```python
from build123d import *

# Parameters (mm, degrees)
SKETCH3_W           = 20
SKETCH3_H           = 60
BOSS_EXTRUDE3_DEPTH = 5
CUT_EXTRUDE2_DEPTH  = 2
SKETCH6_R           = 3.57
CUT_EXTRUDE3_DEPTH  = 3
SKETCH7_W           = 20
SKETCH7_H           = 10
BOSS_EXTRUDE4_DEPTH = 17.5
SKETCH8_R           = 2.1
CUT_EXTRUDE4_DEPTH  = 40
SKETCH9_W           = 1.25
SKETCH9_H           = 25
CUT_EXTRUDE5_DEPTH  = 30


with BuildPart() as part:
    # Sketch3 → Boss-Extrude3 (new body)
    with BuildSketch(Plane.XY):
        Rectangle(SKETCH3_W, SKETCH3_H)
    extrude(amount=BOSS_EXTRUDE3_DEPTH)

    # Sketch4 → Cut-Extrude2 (cut)
    with BuildSketch(Plane.XY.offset(5)):
        with BuildLine():
            Line((-2.85, 19.850023256), (-1.875, 7.739206809))
            Line((-1.875, 7.739206809), (1.875, 7.739206809))
            Line((1.875, 7.739206809), (2.85, 19.850023256))
            ThreePointArc((2.85, 19.850023256), (0, 18.43), (-2.85, 19.850023256))
        make_face()
        with BuildLine():
            Line((1.875, 7.739206809), (-1.875, 7.739206809))
            ThreePointArc((-1.875, 7.739206809), (0, 5.864206809), (1.875, 7.739206809))
        make_face()
        with BuildLine():
            ThreePointArc((3.57, 22), (-1.133666618, 25.385217866), (-2.85, 19.850023256))
            Line((-2.85, 19.850023256), (2.85, 19.850023256))
            ThreePointArc((2.85, 19.850023256), (3.385217866, 20.866333382), (3.57, 22))
        make_face()
        with BuildLine():
            Line((2.85, 19.850023256), (-2.85, 19.850023256))
            ThreePointArc((-2.85, 19.850023256), (0, 18.43), (2.85, 19.850023256))
        make_face()
    extrude(amount=-CUT_EXTRUDE2_DEPTH, mode=Mode.SUBTRACT)

    # Sketch6 → Cut-Extrude3 (cut)
    with BuildSketch(Plane.XY.offset(3)):
        with Locations((0, 22)):
            Circle(SKETCH6_R)
    extrude(amount=-CUT_EXTRUDE3_DEPTH, mode=Mode.SUBTRACT)

    # Sketch7 → Boss-Extrude4 (add)
    with BuildSketch(Plane(origin=(0, 0, 0), x_dir=(-1, 0, 0), z_dir=(0, 0, -1))):
        with Locations((0, -25)):
            Rectangle(SKETCH7_W, SKETCH7_H)
    extrude(amount=BOSS_EXTRUDE4_DEPTH)

    # Sketch8 → Cut-Extrude4 (cut)
    with BuildSketch(Plane(origin=(0, 0, -17.5), x_dir=(-1, 0, 0), z_dir=(0, 0, -1))):
        with Locations((0, -25)):
            Circle(SKETCH8_R)
    extrude(amount=-CUT_EXTRUDE4_DEPTH, mode=Mode.SUBTRACT)

    # Sketch9 → Cut-Extrude5 (cut)
    with BuildSketch(Plane(origin=(10, 0, 0), x_dir=(0, 0, -1), z_dir=(1, 0, 0))):
        with Locations((-0.625, 17.5)):
            Rectangle(SKETCH9_W, SKETCH9_H)
    extrude(amount=-CUT_EXTRUDE5_DEPTH, mode=Mode.SUBTRACT)


solid = part.part
```
Here's how the part is built. I have some questions about the finished solid (model axes, mm). A direction names the side the tool comes from. Round coordinates to 2 decimals unless told otherwise and drop trailing zeros. Order: outer loops, then holes, each group sorted by start corner. A loop starts at its lowest first (then second) coordinate and runs counter-clockwise, first axis right, second up. Notation, with made-up numbers: (-20, 30.25) -> (23, 30.25) arc R21 ccw to (23, 57.25) -> close; hole circle Ø11 at (-2.5, 42). An arc over 180 degrees is marked (long way). Use a Markdown table: item, result. Add a question column.
(1) Suppose I cut it at C-C, the plane y = -25. Please give me the cut outline in (x, z).
(2) For faces 1 (the face through (0, -7, 0)), 2 (the face through (-2.37, 13.88, 4.01)), 3 (the face through (0, 0, 5)), which set-ups out of +Z, -Z, +X, -X, +Y, -Y let a thin tool reach every point of the face, with its end or its side?
(3) If we mould it in two halves opening along Y, with no side actions, what happens to faces 4 (the face through (-1.13, -23.23, -6.41)), 5 (the face through (0, -30, -6)), 6 (the face through (0, -20, -9)), 7 (the face through (10, -14, 1))? For each: released by +Y, released by -Y, zero draft, split by the parting line, or undercut.
(4) I need wall thicknesses on line 1 along Y through (x, z) = (0, 2.55); line 2 along Y through (x, z) = (0, -10.25); line 3 along X through (y, z) = (22, 4.6). Which ranges of each line are inside material? Lowest first, please.
(5) For pin 1 Ø6 at (x, y) = (-2, -10) entering from -Z; pin 2 Ø9 at (x, z) = (0.5, -11) entering from +Y; pin 3 Ø12 at (x, y) = (-1, 15.5) entering from -Z, each with a flat end and sliding along its axis, tell me the tip position at first contact or that it passes through.
(6) Suppose I cut it at A-A, the plane x = 0. Please give me the cut outline in (y, z).
(7) Suppose I cut it at B-B, the plane z = 2. Please give me the cut outline in (x, y).
(8) Suppose I cut it at D-D, the plane z = -5.5. Please give me the cut outline in (x, y), and give its area (3 significant figures).
Verdict:
| question | item | result |
|---|---|---|
| 1 | outline | (-10, -17.5) -> (-2.1, -17.5) -> (-2.1, 5) -> (-10, 5) -> close; (2.1, -17.5) -> (10, -17.5) -> (10, 5) -> (2.1, 5) -> close |
| 2 | face 1 | -Z, +X, -X, +Y |
| 2 | face 2 | +Z |
| 2 | face 3 | +Z, +X, -X, +Y, -Y |
| 3 | face 4 | undercut |
| 3 | face 5 | released by -Y |
| 3 | face 6 | released by +Y |
| 3 | face 7 | zero draft |
| 4 | line 1 | -30 to -27.1, -22.9 to 18.43, 25.57 to 30 |
| 4 | line 2 | -30 to -27.1, -22.9 to -20 |
| 4 | line 3 | -10 to -3.57, 3.57 to 10 |
| 5 | pin 1 | z = 0 |
| 5 | pin 2 | y = -20 |
| 5 | pin 3 | z = 1.25 |
| 6 | outline | (-30, -17.5) -> (-27.1, -17.5) -> (-27.1, 5) -> (-30, 5) -> close; (-22.9, -17.5) -> (-20, -17.5) -> (-20, 0) -> (5, 0) -> (5, 1.25) -> (18.43, 1.25) -> (18.43, 3) -> (5.86, 3) -> (5.86, 5) -> (-22.9, 5) -> close; (25.57, 1.25) -> (30, 1.25) -> (30, 5) -> (25.57, 5) -> close |
| 7 | outline | (-10, -30) -> (10, -30) -> (10, 30) -> (-10, 30) -> close; hole circle Ø7.14 at (0, 22); hole circle Ø4.2 at (0, -25) |
| 8 | outline | (-10, -30) -> (10, -30) -> (10, -20) -> (-10, -20) -> close; hole circle Ø4.2 at (0, -25) |
| 8 | area | 186 mm2 |
